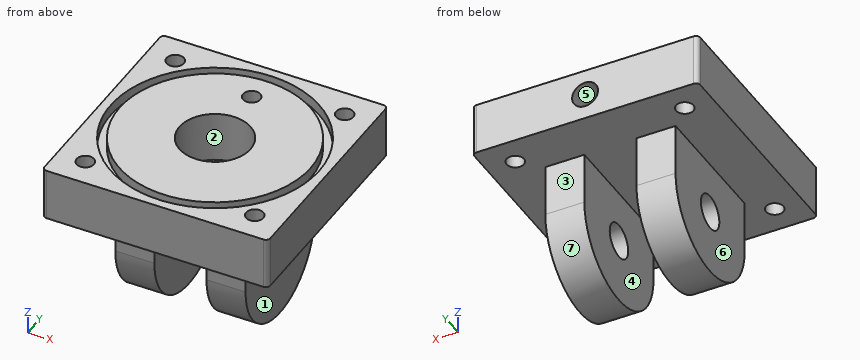
```python
from build123d import *

# Parameters (mm, degrees)
SKETCH1_W                        = 165.1
SKETCH1_H                        = 165.1
BOSS_EXTRUDE1_DEPTH              = 38.1
SKETCH2_W                        = 95.25
SKETCH2_H                        = 95.25
BOSS_EXTRUDE2_DEPTH              = 38.1
BOSS_EXTRUDE3_DEPTH              = 95.25
SKETCH4_R                        = 12.7
CUT_EXTRUDE1_DEPTH               = 177.376894037
SKETCH5_W                        = 38.1
SKETCH5_H                        = 85.725
CUT_EXTRUDE2_DEPTH               = 177.376894037
FILLET1_R                        = 3.175
SKETCH6_R                        = 26
CUT_EXTRUDE3_DEPTH               = 36.83
SKETCH7_R                        = 76.2
SKETCH7_R_2                      = 69.85
CUT_EXTRUDE4_DEPTH               = 8
F_1_2_14_NPSM_TAPPED_HOLE1_D     = 18.9738
F_1_2_14_NPSM_TAPPED_HOLE1_DEPTH = 47.25
F_1_2_14_NPSM_TAPPED_HOLE1_TIP   = 5.700304607
SKETCH11_R                       = 6.35
CUT_EXTRUDE5_DEPTH               = 20
SKETCH12_R                       = 6.35
CUT_EXTRUDE6_DEPTH               = 171.181184746


with BuildPart() as part:
    # Sketch1 → Boss-Extrude1 (new body)
    with BuildSketch(Plane.XY):
        Rectangle(SKETCH1_W, SKETCH1_H)
    extrude(amount=BOSS_EXTRUDE1_DEPTH)

    # Sketch2 → Boss-Extrude2 (add)
    with BuildSketch(Plane(origin=(0, 0, 0), x_dir=(-1, 0, 0), z_dir=(0, 0, -1))):
        Rectangle(SKETCH2_W, SKETCH2_H)
    extrude(amount=BOSS_EXTRUDE2_DEPTH)

    # Sketch3 → Boss-Extrude3 (add)
    with BuildSketch(Plane(origin=(47.625, 0, 0), x_dir=(0, 0, -1), z_dir=(1, 0, 0))):
        with BuildLine():
            Line((38.1, -47.625), (38.1, 47.625))
            ThreePointArc((38.1, 47.625), (85.725, 0), (38.1, -47.625))
        make_face()
    extrude(amount=-BOSS_EXTRUDE3_DEPTH)

    # Sketch4 → Cut-Extrude1 (cut, through all)
    with BuildSketch(Plane(origin=(47.625, 0, 0), x_dir=(0, 0, -1), z_dir=(1, 0, 0))):
        with Locations((38.1, 0)):
            Circle(SKETCH4_R)
    extrude(amount=-CUT_EXTRUDE1_DEPTH, mode=Mode.SUBTRACT)

    # Sketch5 → Cut-Extrude2 (cut, through all)
    with BuildSketch(Plane(origin=(0, 47.625, 0), x_dir=(1, 0, 0), z_dir=(0, 1, 0))):
        with Locations((0, 42.8625)):
            Rectangle(SKETCH5_W, SKETCH5_H)
    extrude(amount=-CUT_EXTRUDE2_DEPTH, mode=Mode.SUBTRACT)

    # Fillet1
    fillet1_edges = [part.edges().sort_by_distance(p)[0] for p in [
        (-82.55, 82.55, 19.05),
        (82.55, 82.55, 19.05),
        (82.55, -82.55, 19.05),
        (-82.55, -82.55, 19.05),
    ]]
    fillet(fillet1_edges, radius=FILLET1_R)

    # Sketch6 → Cut-Extrude3 (cut)
    with BuildSketch(Plane.XY.offset(38.1)):
        Circle(SKETCH6_R)
    extrude(amount=-CUT_EXTRUDE3_DEPTH, mode=Mode.SUBTRACT)

    # Sketch7 → Cut-Extrude4 (cut)
    with BuildSketch(Plane.XY.offset(38.1)):
        Circle(SKETCH7_R)
        Circle(SKETCH7_R_2, mode=Mode.SUBTRACT)
    extrude(amount=-CUT_EXTRUDE4_DEPTH, mode=Mode.SUBTRACT)

    # 1/2-14 NPSM Tapped Hole1
    with Locations(Plane(origin=(0, 82.55, 0), x_dir=(1, 0, 0), z_dir=(0, 1, 0))):
        with Locations((0, -19.05)):
            Hole(F_1_2_14_NPSM_TAPPED_HOLE1_D / 2, depth=F_1_2_14_NPSM_TAPPED_HOLE1_DEPTH)
            with Locations((0, 0, -(F_1_2_14_NPSM_TAPPED_HOLE1_DEPTH + F_1_2_14_NPSM_TAPPED_HOLE1_TIP / 2))):  # 118° drill point
                Cone(0, F_1_2_14_NPSM_TAPPED_HOLE1_D / 2, F_1_2_14_NPSM_TAPPED_HOLE1_TIP, mode=Mode.SUBTRACT)

    # Sketch11 → Cut-Extrude5 (cut)
    with BuildSketch(Plane.XY.offset(38.1)):
        with Locations((0, 50.55)):
            Circle(SKETCH11_R)
    extrude(amount=-CUT_EXTRUDE5_DEPTH, mode=Mode.SUBTRACT)

    # Sketch12 → Cut-Extrude6 (cut, through all)
    with BuildSketch(Plane.XY.offset(38.1)):
        with Locations((-61.963767235, 61.963767235)):
            Circle(SKETCH12_R)
        with Locations((61.963767235, 61.963767235)):
            Circle(SKETCH12_R)
        with Locations((61.963767235, -61.963767235)):
            Circle(SKETCH12_R)
        with Locations((-61.963767235, -61.963767235)):
            Circle(SKETCH12_R)
    extrude(amount=-CUT_EXTRUDE6_DEPTH, mode=Mode.SUBTRACT)


solid = part.part
```
CAD build for the part. Positions are in the model's coordinates, mm. Face numbers are marked on the shaded views. A direction names the side the tool comes from. Give positions to 0.01 mm unless a question says otherwise; leave off trailing zeros. Write each loop counter-clockwise with the first axis right and the second up, starting at its lowest first coordinate (ties: lowest second). Pieces come first, ordered by that corner, then holes. Notation, with made-up numbers: (42.25, -23) -> (101.25, -23) arc R10 ccw to (101.25, -9) -> close; hole circle Ø10 at (75.5, -34.75). An arc over 180 degrees is marked (long way). Write each question's results on one line, items separated by ' | '.
1. Cut at C-C, the plane z = -54. Write the cut outline in (x, y) (3 decimals).
Geometry check:
outline: (-47.625, -44.892) -> (-19.05, -44.892) -> (-19.05, 44.892) -> (-47.625, 44.892) -> close; (19.05, -44.892) -> (47.625, -44.892) -> (47.625, 44.892) -> (19.05, 44.892) -> close
2. Drop flat-ended pins along their axis: P1, Ø4, axis at x = -14.5, y = -24.5, coming from the -Z side; P2, Ø4, axis at y = -2, z = -2.5, coming from the +X side (3 decimals); P3, Ø3, axis at y = 12.5, z = -3.5, coming from the -X side (3 decimals). Give the stop position or say it passes through.
Geometry check:
P1: z = 0 | P2: x = 47.625 | P3: x = -47.625
3. Cut at D-D, the plane z = 14. Give the number of separate pieces and of enclosed holes in the cut face, then the cut area to 3 significant figures.
Geometry check:
separate pieces: 1 | enclosed holes: 5 | area: 23,800 mm²
4. Two-plate mould, pull along X, no slides. Class the marked faces 5, 6 and 7: pulls with the +X half, pulls with the -X half, needs draft (parallel to the pull), parting line crosses it, or undercut.
Geometry check:
face 5: undercut | face 6: pulls with the -X half | face 7: needs draft
5. Wall check: probe 1 along Y at (x, z) = (0, 33); probe 2 along X at (y, z) = (-16.5, -1) (3 decimals); probe 3 along X at (y, z) = (37, 33.5). Give the ranges that are in metal, low to high. Write a range as [from, to].
Geometry check:
probe 1: [-82.55, -76.2], [-69.85, -26], [26, 44.2], [56.9, 69.85], [76.2, 82.55] | probe 2: [-47.625, -19.05], [19.05, 47.625] | probe 3: [-82.55, -66.61], [-59.25, 59.25], [66.61, 82.55]
6. Cut at A-A, the plane z = -5. Write the cut outline in (x, y) (3 decimals), then the cut area to 3 significant figures.
Geometry check:
outline: (-47.625, -47.625) -> (-19.05, -47.625) -> (-19.05, 47.625) -> (-47.625, 47.625) -> close; (19.05, -47.625) -> (47.625, -47.625) -> (47.625, 47.625) -> (19.05, 47.625) -> close | area: 5,440 mm²
7. Cut at B-B, the plane x = 12.5. Write the cut outline in (y, z), then the cut area to 3 significant figures.
Geometry check:
outline: (-82.55, 0) -> (82.55, 0) -> (82.55, 38.1) -> (75.17, 38.1) -> (75.17, 30.1) -> (68.72, 30.1) -> (68.72, 38.1) -> (22.8, 38.1) -> (22.8, 1.27) -> (-22.8, 1.27) -> (-22.8, 38.1) -> (-68.72, 38.1) -> (-68.72, 30.1) -> (-75.17, 30.1) -> (-75.17, 38.1) -> (-82.55, 38.1) -> close | area: 4,510 mm²
8. Which spindle directions (+Z, -Z, +X, -X, +Y, -Y) get a long thin tool onto all of the face, cutting with end or side? Do the marked faces 1, 2, 3 and 4. Say none if no direction does.
Geometry check:
face 1: -Z, +X, +Y, -Y | face 2: +Z | face 3: -Z, +X, -X, +Y | face 4: -Z, +Y, -Y
